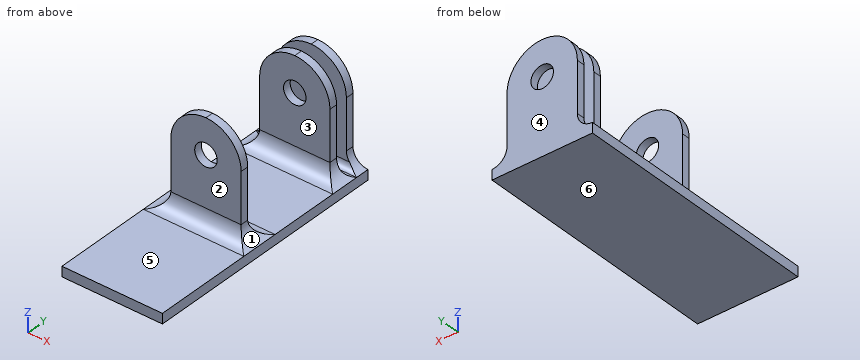
```python
from build123d import *

# Parameters (mm, degrees)
ESQUISSE1_W             = 250
ESQUISSE1_H             = 100
BOSS_EXTRU_1_DEPTH      = 10
ESQUISSE2_W             = 70
ESQUISSE2_H             = 8
BOSS_EXTRU_2_DEPTH      = 100
CONG_1_R                = 35
ESQUISSE3_R             = 11.2
ENL_V_MAT_EXTRU_1_DEPTH = 150
CONG_2_R                = 15
CONG_3_R                = 6


with BuildPart() as part:
    # Esquisse1 → Boss.-Extru.1 (new body)
    with BuildSketch(Plane(origin=(0, 0, 0), x_dir=(0, 1, 0), z_dir=(0, 0, 1))):
        with Locations((125, 50)):
            Rectangle(ESQUISSE1_W, ESQUISSE1_H)
    extrude(amount=BOSS_EXTRU_1_DEPTH)

    # Esquisse2 → Boss.-Extru.2 (add)
    with BuildSketch(Plane.XY.offset(10)):
        with Locations((-50, 226)):
            Rectangle(ESQUISSE2_W, ESQUISSE2_H)
        with Locations((-50, 246)):
            Rectangle(ESQUISSE2_W, ESQUISSE2_H)
        with Locations((-50, 118)):
            Rectangle(ESQUISSE2_W, ESQUISSE2_H)
    extrude(amount=BOSS_EXTRU_2_DEPTH)

    # Congé1
    cong_1_edges = [part.edges().sort_by_distance(p)[0] for p in [
        (-85, 226, 110),
        (-15, 226, 110),
        (-15, 118, 110),
        (-85, 118, 110),
        (-85, 246, 110),
        (-15, 246, 110),
    ]]
    fillet(cong_1_edges, radius=CONG_1_R - 0.0001)  # a hair under: the kernel refuses the full size

    # Esquisse3 → Enlèv. mat.-Extru.1 (cut)
    with BuildSketch(Plane(origin=(0, 250, 0), x_dir=(-1, 0, 0), z_dir=(0, 1, 0))):
        with Locations(Location((50, 75, 0), (0, 0, 90))):
            Circle(ESQUISSE3_R)
    extrude(amount=-ENL_V_MAT_EXTRU_1_DEPTH, mode=Mode.SUBTRACT)

    # Congé2
    cong_2_edges = [part.edges().sort_by_distance(p)[0] for p in [
        (-15, 118, 10),
        (-50, 122, 10),
        (-85, 118, 10),
        (-50, 114, 10),
        (-85, 246, 10),
        (-15, 246, 10),
        (-15, 226, 10),
        (-50, 222, 10),
        (-85, 226, 10),
    ]]
    fillet(cong_2_edges, radius=CONG_2_R - 0.0001)  # a hair under: the kernel refuses the full size

    # Congé3
    cong_3_edges = [part.edges().sort_by_distance(p)[0] for p in [
        (-50, 242, 10),
        (-50, 230, 10),
    ]]
    fillet(cong_3_edges, radius=CONG_3_R - 0.0001)  # a hair under: the kernel refuses the full size


solid = part.part
```
Design review of the part built by this model. Coordinates are the model's own, in mm. Face numbers are marked on the shaded views. A direction names the side the tool comes from. Coordinates: 2 decimals unless noted, no trailing zeros. Order: outer loops, then holes, each group sorted by start corner. A loop starts at its lowest first (then second) coordinate and runs counter-clockwise, first axis right, second up. Notation, with made-up numbers: M 20,-7 L 62,-7 A29 ccw 62,18 Z; hole C -37.75,57 d11. An arc over 180 degrees is marked long. Answer as a JSON object with one key per item and string values. Group by question number.
1) Wall thickness on L1, parallel to Y at x = -35, z = 57; L2, parallel to X at y = 227, z = 75; L3, parallel to Z at x = -6.5, y = 150: over which ranges is each line inside the solid? List them lowest first.
2) For pin 1 (13.5 mm diameter, centred on x = -50, z = 75, fed in from +Y); pin 2 (9 mm diameter, centred on y = 245.5, z = 57.5, fed in from +X); pin 3 (4 mm diameter, centred on x = -81, y = 185.5, fed in from +Z); pin 4 (2.5 mm diameter, centred on y = 116.5, z = 40, fed in from -X), all flat-tipped, find the tip position at first contact; note any pin that passes through.
3) Add section A-A, the plane z = 60.5. Write out the cut boundary in (x, y), then the cut area to 3 significant figures.
4) Add section B-B, the plane x = -46.5. Count the separate pieces of the cut face and the enclosed holes in it, then the cut area to 3 significant figures.
5) Tool access review of the marked faces 1, 2 and 3: name each direction out of +Z, -Z, +X, -X, +Y, -Y from which nothing blocks a thin tool from reaching the whole face with its end or side.
6) Add section C-C, the plane z = 79.5. Write out the cut boundary in (x, y).
7) Add section D-D, the plane y = 200.5. Write out the cut boundary in (x, z), then the cut area to 3 significant figures.
8) Mouldability with a two-part tool opening along Y and no side actions: class the marked faces 4, 5 and 6 as pulls with the +Y half, pulls with the -Y half, needs draft (parallel to the pull), parting line crosses it, or undercut.
Computed values:
{
 "1": {"L1": "y = 114 to 122, 222 to 230, 242 to 250", "L2": "x = -85 to -61.2, -38.8 to -15", "L3": "z = 0 to 10"},
 "2": {"pin 1": "passes through", "pin 2": "stops at x = -15", "pin 3": "stops at z = 10", "pin 4": "stops at x = -85"},
 "3": {"outline": "M -85,114 L -15,114 L -15,122 L -85,122 Z; M -85,222 L -15,222 L -15,230 L -85,230 Z; M -85,242 L -15,242 L -15,250 L -85,250 Z", "area": "1,680 mm^2"},
 "4": {"separate pieces": "4", "enclosed holes": "0", "area": "4,550 mm^2"},
 "5": {"face 1": "+Z, +X, +Y, -Y", "face 2": "+Z, +X, -X, -Y", "face 3": "+Z, +X, -X"},
 "6": {"outline": "M -84.71,114 L -60.26,114 L -60.26,122 L -84.71,122 Z; M -84.71,222 L -60.26,222 L -60.26,230 L -84.71,230 Z; M -84.71,242 L -60.26,242 L -60.26,250 L -84.71,250 Z; M -39.74,114 L -15.29,114 L -15.29,122 L -39.74,122 Z; M -39.74,222 L -15.29,222 L -15.29,230 L -39.74,230 Z; M -39.74,242 L -15.29,242 L -15.29,250 L -39.74,250 Z"},
 "7": {"outline": "M -100,0 L 0,0 L 0,10 L -100,10 Z", "area": "1,000 mm^2"},
 "8": {"face 4": "pulls with the +Y half", "face 5": "undercut", "face 6": "needs draft"}
}
